Here's how the part is built. I have some questions about the finished solid (model axes, mm). Round coordinates to 2 decimals unless told otherwise and drop trailing zeros. Write each loop counter-clockwise with the first axis right and the second up, starting at its lowest first coordinate (ties: lowest second). Pieces come first, ordered by that corner, then holes. Notation, with made-up numbers: (11.5, 66.25) -> (33.5, 66.25) arc R18 cw to (33.5, 82.25) -> close; hole circle Ø4 at (-39.75, 57.25). An arc over 180 degrees is marked (long way). Answer in a Markdown table with one row per item.
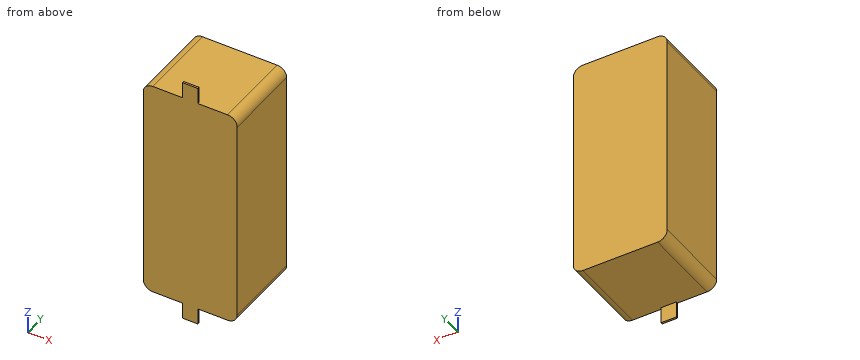
Autodesk Inventor part; units mm, degrees
ref_plane "YZ Plane" through (0, 0, 0) normal (1, 0, 0) x (0, 1, 0)
ref_plane "XZ Plane" through (0, 0, 0) normal (0, 1, 0) x (-1, 0, 0)
ref_plane "XY Plane" through (0, 0, 0) normal (0, 0, 1) x (1, 0, 0)
sketch "Sketch1" plane through (0, 0, 0) normal (0, 1, 0) x (-1, 0, 0)
  line L0 (2.45, 5.8) -> (-2.45, 5.8)
  line L1 (-2.45, 5.8) -> (-2.45, -5.8)
  line L2 (-2.45, -5.8) -> (2.45, -5.8)
  line L3 (2.45, -5.8) -> (2.45, 5.8)
  point P0 (0, 0)
  dimension "d0" = 11.6
  dimension "d1" = 5.8
  dimension "d2" = 4.9
  dimension "d3" = 2.45
extrude "Extrusion1" add sketch "Sketch1" along normal blind 4.2
fillet "Fillet1" radius 0.5 4 edges at (2.45, 2.1, 5.8) (-2.45, 2.1, 5.8) (2.45, 2.1, -5.8) (-2.45, 2.1, -5.8)
sketch "Sketch2" plane through (0, 0, 0) normal (0, -1, 0) x (1, 0, 0)
  line L0 (0.4, 6.65) -> (-0.4, 6.65)
  line L1 (-0.4, 6.65) -> (-0.4, 2.4)
  line L2 (-0.4, 2.4) -> (0.4, 2.4)
  line L3 (0.4, 2.4) -> (0.4, 6.65)
  line L4 (0.4, -2.4) -> (-0.4, -2.4)
  line L5 (-0.4, -2.4) -> (-0.4, -6.65)
  line L6 (-0.4, -6.65) -> (0.4, -6.65)
  line L7 (0.4, -6.65) -> (0.4, -2.4)
  point P0 (0, 0)
  dimension "d7" = 13.3
  dimension "d9" = 4.8
  dimension "d10" = 2.4
  dimension "d11" = 6.65
  dimension "d12" = 0.8
  dimension "d13" = 0.8
  dimension "d14" = 0.4
  dimension "d15" = 0.4
extrude "Extrusion2" add sketch "Sketch2" against normal blind 0.1
properties part number "HC49_XTAL"
1) I want a section at B-B, the plane x = -1.5. List the corners of the cut face in (y, z) for me.
Response:
| item | result |
|---|---|
| outline | (0, -5.8) -> (4.2, -5.8) -> (4.2, 5.8) -> (0, 5.8) -> close |
2) I need wall thicknesses on line 1 (Z direction, x = 1.9, y = 1.1); line 2 (Z direction, x = -2.2, y = 1.35). Which ranges of each line are inside material? Lowest first, please. Write a range as [from, to].
Response:
| item | result |
|---|---|
| line 1 | z = [-5.8, 5.8] |
| line 2 | z = [-5.73, 5.73] |
3) I want a section at A-A, the plane y = 3.95. List the corners of the cut face in (x, z) for me.
Response:
| item | result |
|---|---|
| outline | (-2.45, -5.3) arc R0.5 ccw to (-1.95, -5.8) -> (1.95, -5.8) arc R0.5 ccw to (2.45, -5.3) -> (2.45, 5.3) arc R0.5 ccw to (1.95, 5.8) -> (-1.95, 5.8) arc R0.5 ccw to (-2.45, 5.3) -> close |
4) For pin 1 (2 mm diameter, centred on x = -0.5, y = 2, fed in from +Z); pin 2 (0.6 mm diameter, centred on x = 0, z = -6.5, fed in from +Y), each with a flat end and sliding along its axis, tell me the tip position at first contact or that it passes through.
Response:
| item | result |
|---|---|
| pin 1 | stops at z = 5.8 |
| pin 2 | stops at y = 0.1 |
